```python
from build123d import *

# Parameters (mm, degrees)
SKETCH1_W           = 95
SKETCH1_H           = 55
BOSS_EXTRUDE1_DEPTH = 18
SKETCH2_R           = 4
CUT_EXTRUDE1_DEPTH  = 15
SKETCH3_W           = 35
SKETCH3_H           = 32
CUT_EXTRUDE2_DEPTH  = 12
FILLET2_R           = 2
SKETCH4_W           = 12
SKETCH4_H           = 5
CUT_EXTRUDE3_DEPTH  = 12
SKETCH5_W           = 9
SKETCH5_H           = 5
CUT_EXTRUDE4_DEPTH  = 12


with BuildPart() as part:
    # Sketch1 → Boss-Extrude1 (new body)
    with BuildSketch(Plane(origin=(0, 0, 0), x_dir=(1, 0, 0), z_dir=(0, 1, 0))):
        with Locations((47.5, -27.5)):
            Rectangle(SKETCH1_W, SKETCH1_H)
    extrude(amount=BOSS_EXTRUDE1_DEPTH)

    # Sketch2 → Cut-Extrude1 (cut)
    with BuildSketch(Plane.XY.offset(55)):
        with Locations((80, 9)):
            Circle(SKETCH2_R)
        with Locations((15, 9)):
            Circle(SKETCH2_R)
    extrude(amount=-CUT_EXTRUDE1_DEPTH, mode=Mode.SUBTRACT)

    # Sketch3 → Cut-Extrude2 (cut)
    with BuildSketch(Plane(origin=(0, 18, 0), x_dir=(1, 0, 0), z_dir=(0, 1, 0))):
        with Locations((62, -21)):
            Rectangle(SKETCH3_W, SKETCH3_H)
    extrude(amount=-CUT_EXTRUDE2_DEPTH, mode=Mode.SUBTRACT)

    # Fillet2
    fillet2_edges = [part.edges().sort_by_distance(p)[0] for p in [
        (44.5, 18, 21),
        (62, 18, 37),
        (79.5, 18, 21),
        (62, 18, 5),
        (0, 18, 27.5),
        (0, 0, 27.5),
        (0, 9, 0),
        (0, 9, 55),
    ]]
    fillet(fillet2_edges, radius=FILLET2_R)

    # Sketch4 → Cut-Extrude3 (cut)
    with BuildSketch(Plane(origin=(0, 18, 0), x_dir=(1, 0, 0), z_dir=(0, 1, 0))):
        with Locations((48.5, -2.5)):
            Rectangle(SKETCH4_W, SKETCH4_H)
    extrude(amount=-CUT_EXTRUDE3_DEPTH, mode=Mode.SUBTRACT)

    # Sketch5 → Cut-Extrude4 (cut)
    with BuildSketch(Plane(origin=(0, 18, 0), x_dir=(1, 0, 0), z_dir=(0, 1, 0))):
        with Locations((77, -2.5)):
            Rectangle(SKETCH5_W, SKETCH5_H)
    extrude(amount=-CUT_EXTRUDE4_DEPTH, mode=Mode.SUBTRACT)


solid = part.part
```
Geometry check sheet. Reference: the model listing, model coordinates, mm. A direction names the side the tool comes from. Round coordinates to 2 decimals unless told otherwise and drop trailing zeros. Loops run counter-clockwise (first coordinate to the right, second up) from the corner with the lowest first, then second, coordinate; pieces in that order, holes last. Notation, with made-up numbers: (-31.5, 80.5) - (12.5, 80.5) arc R15 cw to (12.5, 109.5) - close; hole circle Ø2 at (-22, -7). An arc over 180 degrees is marked (long way). Use a Markdown table: item, result.
Q1. Go/stop test with flat-tipped pins: P1, Ø5, axis at x = 76.5, z = 24, coming from the +Y side; P2, Ø1, axis at x = 80.5, y = 9, coming from the -Z side; P3, Ø2.5, axis at x = 78.5, y = 10.5, coming from the +Z side. Record where each tip stops, or that it passes through.
Solutions:
| item | result |
|---|---|
| P1 | stops at y = 6 |
| P2 | stops at z = 5 |
| P3 | stops at z = 40 |
Q2. Cross-section at B-B on x = 15. Record the cut outline in (y, z).
Solutions:
| item | result |
|---|---|
| outline | (0, 0) - (18, 0) - (18, 55) - (13, 55) - (13, 40) - (5, 40) - (5, 55) - (0, 55) - close |
Q3. Material ranges on line 1 (X direction, y = 9.75, z = 14.5); line 2 (Y direction, x = 80, z = 50); line 3 (Z direction, x = 47, y = 16.25), recorded low to high.
Solutions:
| item | result |
|---|---|
| line 1 | x = 0 to 44.5, 79.5 to 95 |
| line 2 | y = 0 to 5, 13 to 18 |
| line 3 | z = 37.02 to 55 |
Q4. Access from +Z, -Z, +X, -X, +Y, -Y to the whole of each face (thin tool, end or side, straight path). Record for faces 1 (the flat face through (62, 11, 37)), 2 (the cylindrical face through (0.57, 17.4, 27.11)), 3 (the cylindrical face through (11, 9, 48)), 4 (the cylindrical face through (0.57, 9.13, 54.4)), 5 (the flat face through (81.5, 12, 3)).
Solutions:
| item | result |
|---|---|
| face 1 | +Y |
| face 2 | +Z, -Z, -X, +Y |
| face 3 | +Z |
| face 4 | +Z, -X, +Y, -Y |
| face 5 | -Z, +Y |
Q5. Cross-section at A-A on y = 9. Record the cut outline in (x, z).
Solutions:
| item | result |
|---|---|
| outline | (0, 2) arc R2 ccw to (2, 0) - (42.5, 0) - (42.5, 5) - (44.5, 5) - (44.5, 37) - (79.5, 37) - (79.5, 5) - (81.5, 5) - (81.5, 0) - (95, 0) - (95, 55) - (84, 55) - (84, 40) - (76, 40) - (76, 55) - (19, 55) - (19, 40) - (11, 40) - (11, 55) - (2, 55) arc R2 ccw to (0, 53) - close; (54.5, 0) - (72.5, 0) - (72.5, 5) - (54.5, 5) - close |
Q6. Cross-section at C-C on z = 19. Record the cut outline in (x, y), plus the area to 3 significant figures.
Solutions:
| item | result |
|---|---|
| outline | (0, 2) arc R2 ccw to (2, 0) - (95, 0) - (95, 18) - (81.5, 18) arc R2 ccw to (79.5, 16) - (79.5, 6) - (44.5, 6) - (44.5, 16) arc R2 ccw to (42.5, 18) - (2, 18) arc R2 ccw to (0, 16) - close |
| area | 1,290 mm2 |
Q7. Draft check along Y on faces 6 (the cylindrical face through (80.1, 17.43, 21.76)), 7 (the cylindrical face through (76, 9, 48)), 8 (the flat face through (44.5, 11, 21)). Enter one of: released by +Y, released by -Y, zero draft, split by the parting line, or undercut.
Solutions:
| item | result |
|---|---|
| face 6 | released by +Y |
| face 7 | undercut |
| face 8 | zero draft |
Q8. Cross-section at D-D on x = 64. Record the cut outline in (y, z), plus the area to 3 significant figures.
Solutions:
| item | result |
|---|---|
| outline | (0, 0) - (18, 0) - (18, 3) arc R2 ccw to (16, 5) - (6, 5) - (6, 37) - (16, 37) arc R2 ccw to (18, 39) - (18, 55) - (0, 55) - close |
| area | 604 mm2 |
